Geometry check sheet. Reference: drawing and pictorial views, mm from the part's lowest x, y, z. A direction names the side the tool comes from. Give positions to 0.01 mm unless a question says otherwise; leave off trailing zeros. Write each loop counter-clockwise with the first axis right and the second up, starting at its lowest first coordinate (ties: lowest second). Pieces come first, ordered by that corner, then holes. Notation, with made-up numbers: M 75,-29 L 94,-29 A23 cw 94,5 Z; hole C -10,57.25 d5. An arc over 180 degrees is marked long. Answer as a JSON object with one key per item and string values.
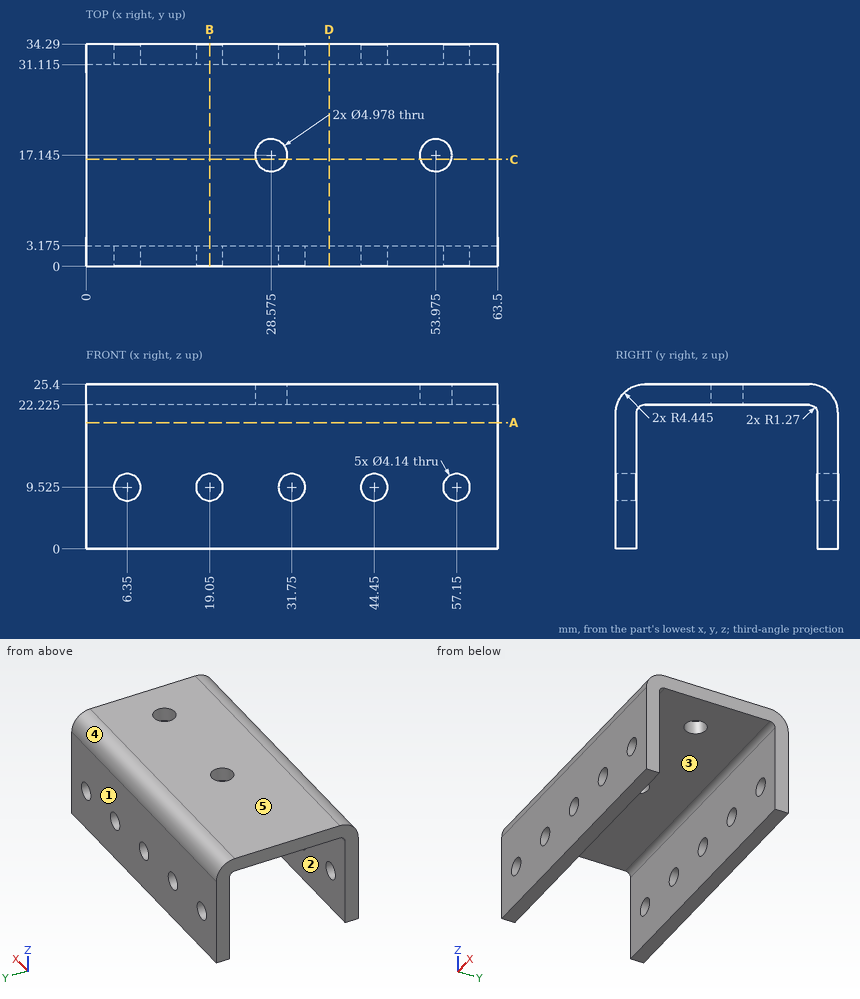
1) Section check C-C on y = 16.5. Record the boundary of the cut face in (x, z) (1 decimal), and give its area (3 significant figures).
Completed:
{"outline": "M 0,22.2 L 26.2,22.2 L 26.2,25.4 L 0,25.4 Z; M 31,22.2 L 51.6,22.2 L 51.6,25.4 L 31,25.4 Z; M 56.4,22.2 L 63.5,22.2 L 63.5,25.4 L 56.4,25.4 Z", "area": "171 mm2"}
2) Thickness scan on L1, parallel to Y at x = 11, z = 10.75 (1 decimal); L2, parallel to Z at x = 37.5, y = 26.5 (1 decimal); L3, parallel to Z at x = 44, y = 32 (1 decimal). Record the ranges inside material, lowest first.
Completed:
{"L1": "y = 0 to 3.2, 31.1 to 34.3", "L2": "z = 22.2 to 25.4", "L3": "z = 0 to 7.5, 11.5 to 24.8"}
3) Section check A-A on z = 19.5. Record the boundary of the cut face in (x, y) (1 decimal), and give its area (3 significant figures).
Completed:
{"outline": "M 0,0 L 63.5,0 L 63.5,3.2 L 0,3.2 Z; M 0,31.1 L 63.5,31.1 L 63.5,34.3 L 0,34.3 Z", "area": "403 mm2"}
4) Section check D-D on x = 37.5. Record the boundary of the cut face in (y, z) (1 decimal), and give its area (3 significant figures).
Completed:
{"outline": "M 0,0 L 3.2,0 L 3.2,21 A1.3 cw 4.4,22.2 L 29.8,22.2 A1.3 cw 31.1,21 L 31.1,0 L 34.3,0 L 34.3,21 A4.4 ccw 29.8,25.4 L 4.4,25.4 A4.4 ccw 0,21 Z", "area": "242 mm2"}
5) Go/stop test with a flat-tipped pin: pin 1 (5.5 mm diameter, centred on x = 28.575, y = 17.145, fed in from -Z) (3 decimals). Record where the tip stops, or that it passes through.
Completed:
{"pin 1": "stops at z = 22.225"}
6) Release check for a two-part mould opening along Y. For the marked faces 3, 4 and 5 record: pulls with the +Y half, pulls with the -Y half, needs draft (parallel to the pull), parting line crosses it, or undercut.
Completed:
{"face 3": "undercut", "face 4": "pulls with the +Y half", "face 5": "needs draft"}
7) Access from +Z, -Z, +X, -X, +Y, -Y to the whole of each face (thin tool, end or side, straight path). Record for the marked faces 1 and 2.
Completed:
{"face 1": "+Z, -Z, +X, -X, +Y", "face 2": "-Z, +X, -X"}
8) Section check B-B on x = 19.05. Record the boundary of the cut face in (y, z) (1 decimal).
Completed:
{"outline": "M 0,0 L 3.2,0 L 3.2,7.5 L 0,7.5 Z; M 0,11.6 L 3.2,11.6 L 3.2,21 A1.3 cw 4.4,22.2 L 29.8,22.2 A1.3 cw 31.1,21 L 31.1,11.6 L 34.3,11.6 L 34.3,21 A4.4 ccw 29.8,25.4 L 4.4,25.4 A4.4 ccw 0,21 Z; M 31.1,0 L 34.3,0 L 34.3,7.5 L 31.1,7.5 Z"}
